```python
from build123d import *

# Parameters (mm, degrees)
SKETCH2_W           = 23
SKETCH2_H           = 42.25
SKETCH2_W_2         = 13
SKETCH2_H_2         = 32.25
BOSS_EXTRUDE1_DEPTH = 20
BOSS_EXTRUDE2_START = -1
SKETCH2_3_R         = 37.5
SKETCH2_3_W         = 23
SKETCH2_3_H         = 42.25
SKETCH2_3_W_2       = 13
SKETCH2_3_H_2       = 32.25
BOSS_EXTRUDE2_DEPTH = 1
SKETCH4_W           = 14
SKETCH4_H           = 5
CUT_EXTRUDE1_DEPTH  = 168


with BuildPart() as part:
    # Sketch2 → Boss-Extrude1 (new body)
    # profile 1 of 5: a face of its own
    with BuildSketch(Plane(origin=(0, 0, 0), x_dir=(1, 0, 0), z_dir=(0, 1, 0))):
        with Locations((6.5, 16.125)):
            Rectangle(SKETCH2_W, SKETCH2_H)
        with Locations((6.5, 16.125)):
            Rectangle(SKETCH2_W_2, SKETCH2_H_2, mode=Mode.SUBTRACT)
    # profile 2 of 5: a face of its own
    with BuildSketch(Plane(origin=(0, 0, 0), x_dir=(1, 0, 0), z_dir=(0, 1, 0))):
        with BuildLine():
            Line((6.5, 1.286), (6.5, 0))
            Line((6.5, 0), (13, 0))
            Line((13, 0), (13, 4))
            Line((13, 4), (6.5, 4))
            Line((6.5, 4), (6.5, 3.286))
            ThreePointArc((6.5, 3.286), (7.207106781, 2.993106781), (7.5, 2.286))
            ThreePointArc((7.5, 2.286), (7.207106781, 1.578893219), (6.5, 1.286))
        make_face()
    # profile 3 of 5: a face of its own
    with BuildSketch(Plane(origin=(0, 0, 0), x_dir=(1, 0, 0), z_dir=(0, 1, 0))):
        with BuildLine():
            Line((0, 4), (0, 0))
            Line((0, 0), (6.5, 0))
            Line((6.5, 0), (6.5, 1.286))
            ThreePointArc((6.5, 1.286), (5.5, 2.286), (6.5, 3.286))
            Line((6.5, 3.286), (6.5, 4))
            Line((6.5, 4), (0, 4))
        make_face()
    # profile 4 of 5: a face of its own
    with BuildSketch(Plane(origin=(0, 0, 0), x_dir=(1, 0, 0), z_dir=(0, 1, 0))):
        with BuildLine():
            Line((6.5, 28.964), (6.5, 28.25))
            Line((6.5, 28.25), (13, 28.25))
            Line((13, 28.25), (13, 32.25))
            Line((13, 32.25), (6.5, 32.25))
            Line((6.5, 32.25), (6.5, 30.964))
            ThreePointArc((6.5, 30.964), (7.207106781, 30.671106781), (7.5, 29.964))
            ThreePointArc((7.5, 29.964), (7.207106781, 29.256893219), (6.5, 28.964))
        make_face()
    # profile 5 of 5: a face of its own
    with BuildSketch(Plane(origin=(0, 0, 0), x_dir=(1, 0, 0), z_dir=(0, 1, 0))):
        with BuildLine():
            Line((0, 32.25), (0, 28.25))
            Line((0, 28.25), (6.5, 28.25))
            Line((6.5, 28.25), (6.5, 28.964))
            ThreePointArc((6.5, 28.964), (5.5, 29.964), (6.5, 30.964))
            Line((6.5, 30.964), (6.5, 32.25))
            Line((6.5, 32.25), (0, 32.25))
        make_face()
    extrude(amount=BOSS_EXTRUDE1_DEPTH)

    # Sketch2_3 → Boss-Extrude2 (add)
    # profile 1 of 13: a face of its own
    with BuildSketch(Plane(origin=(0, 0, 0), x_dir=(1, 0, 0), z_dir=(0, 1, 0)).offset(BOSS_EXTRUDE2_START)):
        with Locations(Location((6.5, 16.125, 0), (0, 0, 270))):
            Circle(SKETCH2_3_R)
        with Locations((6.5, 16.125)):
            Rectangle(SKETCH2_3_W, SKETCH2_3_H, mode=Mode.SUBTRACT)
    # profile 2 of 13: a face of its own
    with BuildSketch(Plane(origin=(0, 0, 0), x_dir=(1, 0, 0), z_dir=(0, 1, 0)).offset(BOSS_EXTRUDE2_START)):
        with Locations((6.5, 16.125)):
            Rectangle(SKETCH2_3_W, SKETCH2_3_H)
        with Locations((6.5, 16.125)):
            Rectangle(SKETCH2_3_W_2, SKETCH2_3_H_2, mode=Mode.SUBTRACT)
    # profile 3 of 13: a face of its own
    with BuildSketch(Plane(origin=(0, 0, 0), x_dir=(1, 0, 0), z_dir=(0, 1, 0)).offset(BOSS_EXTRUDE2_START)):
        Polygon((0, 28.25), (0, 4), (6.5, 4), (13, 4), (13, 28.25), (6.5, 28.25), align=None)
    # profile 4 of 13: a face of its own
    with BuildSketch(Plane(origin=(0, 0, 0), x_dir=(1, 0, 0), z_dir=(0, 1, 0)).offset(BOSS_EXTRUDE2_START)):
        with BuildLine():
            Line((6.5, 28.964), (6.5, 28.25))
            Line((6.5, 28.25), (13, 28.25))
            Line((13, 28.25), (13, 32.25))
            Line((13, 32.25), (6.5, 32.25))
            Line((6.5, 32.25), (6.5, 30.964))
            ThreePointArc((6.5, 30.964), (7.207106781, 30.671106781), (7.5, 29.964))
            ThreePointArc((7.5, 29.964), (7.207106781, 29.256893219), (6.5, 28.964))
        make_face()
    # profile 5 of 13: a face of its own
    with BuildSketch(Plane(origin=(0, 0, 0), x_dir=(1, 0, 0), z_dir=(0, 1, 0)).offset(BOSS_EXTRUDE2_START)):
        with BuildLine():
            ThreePointArc((6.5, 30.964), (5.5, 29.964), (6.5, 28.964))
            Line((6.5, 28.964), (6.5, 29.964))
            Line((6.5, 29.964), (6.5, 30.964))
        make_face()
    # profile 6 of 13: a face of its own
    with BuildSketch(Plane(origin=(0, 0, 0), x_dir=(1, 0, 0), z_dir=(0, 1, 0)).offset(BOSS_EXTRUDE2_START)):
        with BuildLine():
            Line((6.5, 29.964), (6.5, 28.964))
            ThreePointArc((6.5, 28.964), (7.207106781, 29.256893219), (7.5, 29.964))
            ThreePointArc((7.5, 29.964), (7.207106781, 30.671106781), (6.5, 30.964))
            Line((6.5, 30.964), (6.5, 29.964))
        make_face()
    # profile 7 of 13: a face of its own
    with BuildSketch(Plane(origin=(0, 0, 0), x_dir=(1, 0, 0), z_dir=(0, 1, 0)).offset(BOSS_EXTRUDE2_START)):
        with BuildLine():
            Line((0, 32.25), (0, 28.25))
            Line((0, 28.25), (6.5, 28.25))
            Line((6.5, 28.25), (6.5, 28.964))
            ThreePointArc((6.5, 28.964), (5.5, 29.964), (6.5, 30.964))
            Line((6.5, 30.964), (6.5, 32.25))
            Line((6.5, 32.25), (0, 32.25))
        make_face()
    # profile 8 of 13: a face of its own
    with BuildSketch(Plane(origin=(0, 0, 0), x_dir=(1, 0, 0), z_dir=(0, 1, 0)).offset(BOSS_EXTRUDE2_START)):
        with BuildLine():
            ThreePointArc((6.5, 30.964), (5.5, 29.964), (6.5, 28.964))
            Line((6.5, 28.964), (6.5, 29.964))
            Line((6.5, 29.964), (6.5, 30.964))
        make_face()
    # profile 9 of 13: a face of its own
    with BuildSketch(Plane(origin=(0, 0, 0), x_dir=(1, 0, 0), z_dir=(0, 1, 0)).offset(BOSS_EXTRUDE2_START)):
        with BuildLine():
            Line((6.5, 29.964), (6.5, 28.964))
            ThreePointArc((6.5, 28.964), (7.207106781, 29.256893219), (7.5, 29.964))
            ThreePointArc((7.5, 29.964), (7.207106781, 30.671106781), (6.5, 30.964))
            Line((6.5, 30.964), (6.5, 29.964))
        make_face()
    # profile 10 of 13: a face of its own
    with BuildSketch(Plane(origin=(0, 0, 0), x_dir=(1, 0, 0), z_dir=(0, 1, 0)).offset(BOSS_EXTRUDE2_START)):
        with BuildLine():
            Line((6.5, 1.286), (6.5, 0))
            Line((6.5, 0), (13, 0))
            Line((13, 0), (13, 4))
            Line((13, 4), (6.5, 4))
            Line((6.5, 4), (6.5, 3.286))
            ThreePointArc((6.5, 3.286), (7.207106781, 2.993106781), (7.5, 2.286))
            ThreePointArc((7.5, 2.286), (7.207106781, 1.578893219), (6.5, 1.286))
        make_face()
    # profile 11 of 13: a face of its own
    with BuildSketch(Plane(origin=(0, 0, 0), x_dir=(1, 0, 0), z_dir=(0, 1, 0)).offset(BOSS_EXTRUDE2_START)):
        with BuildLine():
            Line((0, 4), (0, 0))
            Line((0, 0), (6.5, 0))
            Line((6.5, 0), (6.5, 1.286))
            ThreePointArc((6.5, 1.286), (5.5, 2.286), (6.5, 3.286))
            Line((6.5, 3.286), (6.5, 4))
            Line((6.5, 4), (0, 4))
        make_face()
    # profile 12 of 13: a face of its own
    with BuildSketch(Plane(origin=(0, 0, 0), x_dir=(1, 0, 0), z_dir=(0, 1, 0)).offset(BOSS_EXTRUDE2_START)):
        with BuildLine():
            ThreePointArc((6.5, 3.286), (5.5, 2.286), (6.5, 1.286))
            Line((6.5, 1.286), (6.5, 2.286))
            Line((6.5, 2.286), (6.5, 3.286))
        make_face()
    # profile 13 of 13: a face of its own
    with BuildSketch(Plane(origin=(0, 0, 0), x_dir=(1, 0, 0), z_dir=(0, 1, 0)).offset(BOSS_EXTRUDE2_START)):
        with BuildLine():
            Line((6.5, 2.286), (6.5, 1.286))
            ThreePointArc((6.5, 1.286), (7.207106781, 1.578893219), (7.5, 2.286))
            ThreePointArc((7.5, 2.286), (7.207106781, 2.993106781), (6.5, 3.286))
            Line((6.5, 3.286), (6.5, 2.286))
        make_face()
    extrude(amount=BOSS_EXTRUDE2_DEPTH)

    # Sketch4 → Cut-Extrude1 (cut)
    with BuildSketch(Plane(origin=(0, 0, -37.25), x_dir=(-1, 0, 0), z_dir=(0, 0, -1))):
        with Locations((-7, 2.5)):
            Rectangle(SKETCH4_W, SKETCH4_H)
    extrude(amount=-CUT_EXTRUDE1_DEPTH, mode=Mode.SUBTRACT)


solid = part.part
```
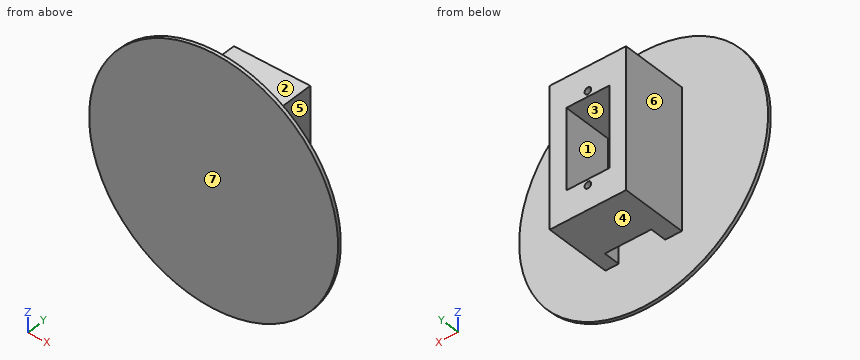
CAD build for the part. Positions are in the model's coordinates, mm. Face numbers are marked on the shaded views. A direction names the side the tool comes from. Round coordinates to 2 decimals unless told otherwise and drop trailing zeros. Loops run counter-clockwise (first coordinate to the right, second up) from the corner with the lowest first, then second, coordinate; pieces in that order, holes last. Notation, with made-up numbers: M -11,66.25 L 26,66.25 A15 cw 26,72.25 Z; hole C 30.25,68.5 d7. An arc over 180 degrees is marked long. Return JSON: item names as keys, results as strings. Group by question number.
(1) Tool access for the marked faces 5, 6 and 7: list every direction of +Z, -Z, +X, -X, +Y, -Y with a clear straight run to the whole face (end or side of a thin tool).
(2) Saw through at B-B, the plane y = 15. List the corners of the cut face in (x, z).
(3) Mould opens along Z. For the marked faces 1, 2, 3 and 4 say: +Z half, -Z half, draft (parallel to the pull), parting line (faces both ways), or undercut.
(4) Drop flat-ended pins along their axis: P1, Ø6, axis at y = 12.5, z = -12, coming from the +X side; P2, Ø10.5, axis at x = 8, y = 14, coming from the -Z side; P3, Ø4.5, axis at y = 9.5, z = -19, coming from the -X side. Give the stop position or say it passes through.
(5) Saw through at A-A, the plane y = 3. List the corners of the cut face in (x, z), and give its area (3 significant figures).
(6) Saw through at C-C, the plane x = 9. List the corners of the cut face in (y, z).
(7) Wall check: probe 1 along X at (y, z) = (6.5, -25); probe 2 along X at (y, z) = (4.5, -23); probe 3 along Z at (x, y) = (4, 14.25). Give the ranges that are in metal, low to high. Write a range as [from, to].
(8) Saw through at D-D, the plane z = -13.5. List the corners of the cut face in (x, y), and give its area (3 significant figures).
Answer list:
{
 "1": {"face 5": "+Z, -Z, +X, +Y", "face 6": "+Z, -Z, -X, +Y", "face 7": "+Z, -Z, +X, -X, -Y"},
 "2": {"outline": "M -5,-37.25 L 18,-37.25 L 18,5 L -5,5 Z; hole M 0,-28.25 L 13,-28.25 L 13,-4 L 0,-4 Z; hole C 6.5,-29.96 d2; hole C 6.5,-2.29 d2"},
 "3": {"face 1": "undercut", "face 2": "+Z half", "face 3": "undercut", "face 4": "-Z half"},
 "4": {"P1": "x = 18", "P2": "z = -37.25", "P3": "x = -5"},
 "5": {"outline": "M -5,-37.25 L 0,-37.25 L 0,5 L -5,5 Z; M 14,-37.25 L 18,-37.25 L 18,5 L 14,5 Z", "area": "380 mm2"},
 "6": {"outline": "M -1,-53.54 L 0,-53.54 L 0,21.29 L -1,21.29 Z; M 5,-37.25 L 20,-37.25 L 20,-28.25 L 5,-28.25 Z; M 5,-4 L 20,-4 L 20,5 L 5,5 Z"},
 "7": {"probe 1": "[-5, 0], [13, 18]", "probe 2": "[-5, 0], [14, 18]", "probe 3": "[-37.25, -28.25], [-4, 5]"},
 "8": {"outline": "M -30.91,-1 L 43.91,-1 L 43.91,0 L 18,0 L 18,20 L 13,20 L 13,5 L 14,5 L 14,0 L 0,0 L 0,20 L -5,20 L -5,0 L -30.91,0 Z", "area": "270 mm2"}
}
